from build123d import *

# Parameters (mm, degrees)
BASE_FLANGE1_DEPTH = 1


# Sheet-metal steps are written as plain solids
with BuildPart() as part:
    # Sketch1 → Base-Flange1 (new body)
    with BuildSketch(Plane.XY):
        with BuildLine():
            Line((42.5, 4.5), (42.5, 0))
            Line((42.5, 0), (1.5, 0))
            ThreePointArc((1.5, 0), (1.060660172, 1.060660172), (0, 1.5))
            Line((0, 1.5), (0, 20.5))
            Line((0, 20.5), (26.5, 20.5))
            ThreePointArc((26.5, 20.5), (37.813708499, 15.813708499), (42.5, 4.5))
        make_face()
    extrude(amount=-BASE_FLANGE1_DEPTH)


solid = part.part
For this review, take the finished solid that the model builds, in its own axes (mm). Give positions to 0.01 mm unless a question says otherwise; leave off trailing zeros. Loops run counter-clockwise (first coordinate to the right, second up) from the corner with the lowest first, then second, coordinate; pieces in that order, holes last. Notation, with made-up numbers: (79.25, -1.5) -> (91.25, -1.5) arc R26 ccw to (91.25, 13.5) -> close; hole circle Ø2 at (-18, -29.75). An arc over 180 degrees is marked (long way). One line per question, with ' | ' between items.
1) We need section B-B (y = 16.5). Write out the cut boundary in (x, z), plus the area to 3 significant figures.
Resolved:
outline: (0, -1) -> (37.08, -1) -> (37.08, 0) -> (0, 0) -> close | area: 37.1 mm2
2) We need section C-C (x = 35). Write out the cut boundary in (y, z), plus the area to 3 significant figures.
Resolved:
outline: (0, -1) -> (18.06, -1) -> (18.06, 0) -> (0, 0) -> close | area: 18.1 mm2
3) To check wall thickness, follow probe 1 along X at (y, z) = (14.5, -0.8); probe 2 along X at (y, z) = (7.5, -0.6); probe 3 along Y at (x, z) = (35, -0.1). State the ranges of each line that lie inside material, in increasing order.
Resolved:
probe 1: x = 0 to 38.99 | probe 2: x = 0 to 42.22 | probe 3: y = 0 to 18.06
4) We need section A-A (z = -0.85). Write out the cut boundary in (x, y), plus the area to 3 significant figures.
Resolved:
outline: (0, 1.5) arc R1.5 cw to (1.5, 0) -> (42.5, 0) -> (42.5, 4.5) arc R16 ccw to (26.5, 20.5) -> (0, 20.5) -> close | area: 815 mm2
